from build123d import *

# Parameters (mm, degrees)
F1_DEPTH = 50
F2_W     = 19.9999988079
F2_H     = 30
F3_DEPTH = 70


with BuildPart() as f1:
    # F0 (on Top) → F1 (new body)
    with BuildSketch(Plane.XY):
        Polygon((-48.3720720015, 10), (-48.3720720015, 0), (-8.3720720015, 0), (-8.3720720015, 20), (31.6279279985, 20), (31.6279279985, 0), (71.6279279985, 0), (71.6279279985, 10), (46.6279279985, 10), (46.6279279985, 50), (26.6279279985, 50), (26.6279279985, 40), (-3.3720720015, 40), (-3.3720720015, 50), (-23.3720720015, 50), (-23.3720720015, 10), align=None)
    extrude(amount=F1_DEPTH)

    # F2 (on face) → F3 (cut)
    with BuildSketch(Plane.YZ.offset(46.6279279985)):
        with Locations((40.000000596, 24.4267614186)):
            Rectangle(F2_W, F2_H)
    extrude(amount=-F3_DEPTH, mode=Mode.SUBTRACT)


solid = f1.part
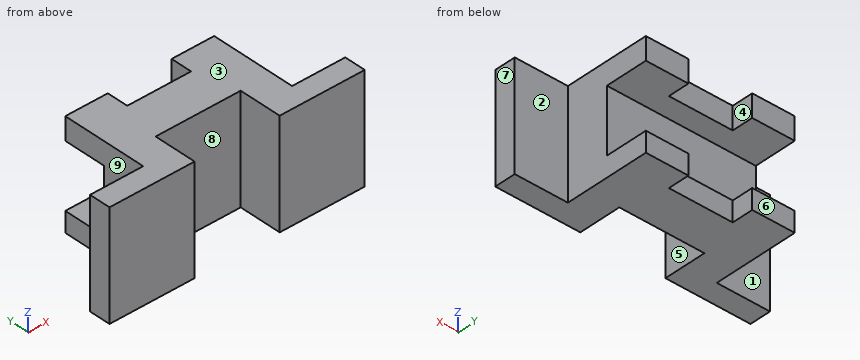
Design review of the part built by this model. Coordinates are the model's own, in mm. Face numbers are marked on the shaded views. A direction names the side the tool comes from. Coordinates: 2 decimals unless noted, no trailing zeros. Order: outer loops, then holes, each group sorted by start corner. A loop starts at its lowest first (then second) coordinate and runs counter-clockwise, first axis right, second up.
Item 1: For the marked faces 1, 2, 3, 4 and 5, list the 3-axis set-ups (+Z, -Z, +X, -X, +Y, -Y) from which the entire face can be reached by the end or side of a thin tool; tool diameter is ignored.
Item 2: Take a section at B-B, the plane x = -12.5. Write out the cut boundary in (y, z), then the cut area to 3 significant figures.
Item 3: For pin 1 Ø7.5 at (y, z) = (46, 6.5) entering from -X; pin 2 Ø4.5 at (y, z) = (43.5, 5) entering from +X; pin 3 Ø12.5 at (x, z) = (-34.5, 18) entering from +Y; pin 4 Ø10 at (x, y) = (-3, 7.5) entering from -Z, all flat-tipped, find the tip position at first contact; note any pin that passes through.
Item 4: Take a section at A-A, the plane y = 14. Write out the cut boundary in (x, z), then the cut area to 3 significant figures.
Item 5: Take a section at D-D, the plane y = 44. Write out the cut boundary in (x, z).
Item 6: Take a section at C-C, the plane z = 44.5. Write out the cut boundary in (x, y), then the cut area to 3 significant figures.
Item 7: For line 1 (X direction, y = 7.5, z = 33.5); line 2 (Z direction, x = -17, y = 43); line 3 (X direction, y = 43, z = 41.5), list the stretches that pass through material, from the lowest coordinate up.
Item 8: The part is to be moulded in two halves that separate along X. For the marked faces 6, 7, 8 and 9, say which applies: pulls with the +X half, pulls with the -X half, needs draft (parallel to the pull), parting line crosses it, or undercut.
The answers:
1. face 1: +Z, -Z, -X, +Y
1. face 2: +Z, -Z, +X, +Y
1. face 3: +Z, +X, -X, +Y, -Y
1. face 4: +Z, -Z, +Y
1. face 5: +Z, -Z, -Y
2. outline: (0, 0) - (50, 0) - (50, 9.43) - (30, 9.43) - (30, 39.43) - (50, 39.43) - (50, 50) - (0, 50) - close
2. area: 1,900 mm2
3. pin 1: stops at x = -23.37
3. pin 2: stops at x = 46.63
3. pin 3: stops at y = 10
3. pin 4: passes through
4. outline: (-23.37, 0) - (-8.37, 0) - (-8.37, 50) - (-23.37, 50) - close; (31.63, 0) - (46.63, 0) - (46.63, 50) - (31.63, 50) - close
4. area: 1,500 mm2
5. outline: (-23.37, 0) - (-3.37, 0) - (-3.37, 9.43) - (-23.37, 9.43) - close; (-23.37, 39.43) - (-3.37, 39.43) - (-3.37, 50) - (-23.37, 50) - close; (26.63, 0) - (46.63, 0) - (46.63, 9.43) - (26.63, 9.43) - close; (26.63, 39.43) - (46.63, 39.43) - (46.63, 50) - (26.63, 50) - close
6. outline: (-48.37, 0) - (-8.37, 0) - (-8.37, 20) - (31.63, 20) - (31.63, 0) - (71.63, 0) - (71.63, 10) - (46.63, 10) - (46.63, 50) - (26.63, 50) - (26.63, 40) - (-3.37, 40) - (-3.37, 50) - (-23.37, 50) - (-23.37, 10) - (-48.37, 10) - close
6. area: 2,900 mm2
7. line 1: x = -48.37 to -8.37, 31.63 to 71.63
7. line 2: z = 0 to 9.43, 39.43 to 50
7. line 3: x = -23.37 to -3.37, 26.63 to 46.63
8. face 6: needs draft
8. face 7: pulls with the +X half
8. face 8: undercut
8. face 9: pulls with the -X half
